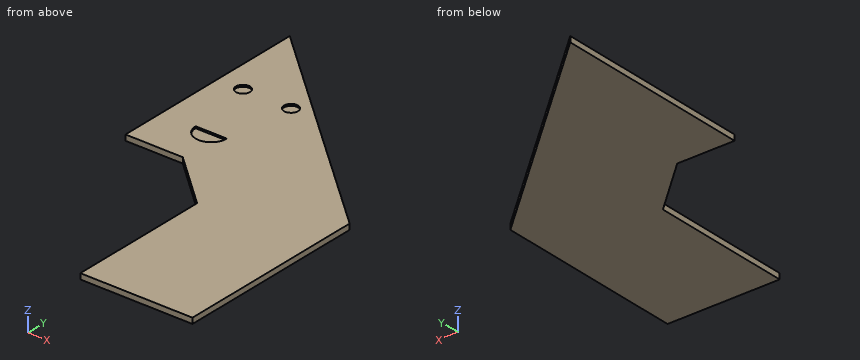
```python
from build123d import *

# Parameters (mm, degrees)
F1_DEPTH = 2.5
F3_R     = 3.175
F4_DEPTH = 0.79375


with BuildPart() as f1:
    # F0 (on Top) → F1 (new body)
    with BuildSketch(Plane.XY):
        Polygon((0, 90), (0, 0), (25.572903, 0), (50, -22.149762), (50, -86.09388), (100, -86.09388), (100, 0), align=None)
    extrude(amount=F1_DEPTH)

    # F3 (on face) → F4 (cut)
    with BuildSketch(Plane.XY.offset(2.5)):
        with BuildLine():
            Line((29.080364, 19.845134), (15.167672, 19.845134))
            ThreePointArc((15.167672, 19.845134), (22.124018, 12.888788), (29.080364, 19.845134))
        make_face()
        with Locations((11.280774, 50.523829)):
            Circle(F3_R)
        with Locations((32.720824, 50.523829)):
            Circle(F3_R)
    extrude(amount=-F4_DEPTH, mode=Mode.SUBTRACT)


solid = f1.part
```
CAD build for the part. Positions are in the model's coordinates, mm. Round coordinates to 2 decimals unless told otherwise and drop trailing zeros. Loops run counter-clockwise (first coordinate to the right, second up) from the corner with the lowest first, then second, coordinate; pieces in that order, holes last. Notation, with made-up numbers: M -36.5,89 L 5.5,89 A29 ccw 5.5,111 Z; hole C 46.25,46 d5. An arc over 180 degrees is marked long. Use a Markdown table: item, result. Add a question column.
(1) Cut at C-C (y = -70.5). Give the cut face in (x, z), and give its area (3 significant figures).
(2) Cut at A-A (z = 0.4). Give the cut face in (x, y), and give its area (3 significant figures).
(3) Drill centre lines: line 1 (Y direction, x = 34, z = 2.25); line 2 (X direction, y = -65, z = 1.65); line 3 (X direction, y = 18, z = 2). Where is each one in solid material? Low to high.
(4) Cut at B-B (x = 69). Give the cut face in (y, z).
(5) Flat gauge pins, fed straight in: pin 1 (0.8 mm diameter, centred on x = 7, z = 0.5, fed in from -Y); pin 2 (3 mm diameter, centred on x = 31.5, y = 51, fed in from +Z); pin 3 (0.8 mm diameter, centred on y = -41.5, z = 2, fed in from -X). Where does each tip first touch, or does it go through?
(6) Cut at D-D (x = 33). Give the cut face in (y, z), and give its area (3 significant figures).
Geometry says:
| question | item | result |
|---|---|---|
| 1 | outline | M 50,0 L 100,0 L 100,2.5 L 50,2.5 Z |
| 1 | area | 125 mm² |
| 2 | outline | M 0,0 L 25.57,0 L 50,-22.15 L 50,-86.09 L 100,-86.09 L 100,0 L 0,90 Z |
| 2 | area | 9,080 mm² |
| 3 | line 1 | y = -7.64 to 47.62, 53.43 to 59.4 |
| 3 | line 2 | x = 50 to 100 |
| 3 | line 3 | x = 0 to 15.42, 28.83 to 80 |
| 4 | outline | M -86.09,0 L 27.9,0 L 27.9,2.5 L -86.09,2.5 Z |
| 5 | pin 1 | stops at y = 0 |
| 5 | pin 2 | stops at z = 1.71 |
| 5 | pin 3 | stops at x = 50 |
| 6 | outline | M -6.73,0 L 60.3,0 L 60.3,2.5 L 53.69,2.5 L 53.69,1.71 L 47.36,1.71 L 47.36,2.5 L -6.73,2.5 Z |
| 6 | area | 163 mm² |
